from build123d import *

# Parameters (mm, degrees)
CROQUIS1_W              = 64
CROQUIS1_H              = 64
SALIENTE_EXTRUIR1_DEPTH = 60
CROQUIS2_W              = 70
CROQUIS2_H              = 70
CROQUIS2_W_2            = 64
CROQUIS2_H_2            = 64
SALIENTE_EXTRUIR2_DEPTH = 64
CORTAR_EXTRUIR1_DEPTH   = 21
CROQUIS5_R              = 1.1
CORTAR_EXTRUIR2_DEPTH   = 10
CORTAR_EXTRUIR3_REACH   = 30
CROQUIS10_R             = 4.5
CROQUIS11_W             = 70
CROQUIS11_H             = 70
CORTAR_EXTRUIR4_DEPTH   = 30
CROQUIS12_W             = 23
CROQUIS12_H             = 12.2
CORTAR_EXTRUIR5_DEPTH   = 21
CORTAR_EXTRUIR6_REACH   = 30
CROQUIS13_R             = 4.5
CROQUIS14_R             = 1.1
CORTAR_EXTRUIR7_DEPTH   = 10
CROQUIS15_R             = 3.7
CORTAR_EXTRUIR8_DEPTH   = 10
CROQUIS16_W             = 64
CROQUIS16_H             = 64
CORTAR_EXTRUIR9_DEPTH   = 5
CROQUIS17_W             = 12.5
CROQUIS17_H             = 12.998685397
CORTAR_EXTRUIR10_DEPTH  = 5
CORTAR_EXTRUIR11_REACH  = 72
CROQUIS18_W             = 70
CROQUIS18_H             = 9
CROQUIS18_H_2           = 5.000169364
CORTAR_EXTRUIR13_DEPTH  = 5
CORTAR_EXTRUIR14_REACH  = 12
CROQUIS21_W             = 81.467019472
CROQUIS21_H             = 81.467019472
CORTAR_EXTRUIR15_REACH  = 5
CROQUIS22_W             = 3.1
CROQUIS22_H             = 12.2


with BuildPart() as part:
    # Croquis1 → Saliente-Extruir1 (new body)
    with BuildSketch(Plane(origin=(0, 0, 0), x_dir=(1, 0, 0), z_dir=(0, 1, 0))):
        Rectangle(CROQUIS1_W, CROQUIS1_H)
    extrude(amount=SALIENTE_EXTRUIR1_DEPTH)

    # Croquis2 → Saliente-Extruir2 (add)
    with BuildSketch(Plane(origin=(0, 0, 0), x_dir=(1, 0, 0), z_dir=(0, 1, 0))):
        Rectangle(CROQUIS2_W, CROQUIS2_H)
        Rectangle(CROQUIS2_W_2, CROQUIS2_H_2, mode=Mode.SUBTRACT)
    extrude(amount=SALIENTE_EXTRUIR2_DEPTH)

    # Croquis4 → Cortar-Extruir1 (cut)
    with BuildSketch(Plane(origin=(0, 60, 0), x_dir=(1, 0, 0), z_dir=(0, 1, 0))):
        Polygon((-7, 6), (-7, -6), (-7, -6.25), (16, -6.25), (16, -6), (16, 6), (16, 6.25), (-7, 6.25), align=None)
    extrude(amount=-CORTAR_EXTRUIR1_DEPTH, mode=Mode.SUBTRACT)

    # Croquis5 → Cortar-Extruir2 (cut)
    with BuildSketch(Plane(origin=(0, 60, 0), x_dir=(1, 0, 0), z_dir=(0, 1, 0))):
        with Locations((19, 0)):
            Circle(CROQUIS5_R)
        with Locations((-9, 0)):
            Circle(CROQUIS5_R)
    extrude(amount=-CORTAR_EXTRUIR2_DEPTH, mode=Mode.SUBTRACT)

    # Croquis10 → Cortar-Extruir3 (cut, up to next)
    with BuildSketch(Plane(origin=(-7, 0, 0), x_dir=(0, 0, -1), z_dir=(1, 0, 0)), mode=Mode.PRIVATE) as cortar_extruir3_sk1:
        with Locations((0, 44)):
            Circle(CROQUIS10_R)
    cortar_extruir3_tool1 = extrude(cortar_extruir3_sk1.sketch, amount=-CORTAR_EXTRUIR3_REACH, mode=Mode.PRIVATE) & part.part
    add(cortar_extruir3_tool1.solids().sort_by_distance((-7, 44, 0))[0], mode=Mode.SUBTRACT)

    # Croquis11 → Cortar-Extruir4 (cut)
    with BuildSketch(Plane.XZ):
        Rectangle(CROQUIS11_W, CROQUIS11_H)
    extrude(amount=-CORTAR_EXTRUIR4_DEPTH, mode=Mode.SUBTRACT)

    # Croquis12 → Cortar-Extruir5 (cut)
    with BuildSketch(Plane.XZ.offset(-30)):
        with Locations((4.5, 22.1)):
            Rectangle(CROQUIS12_W, CROQUIS12_H)
    extrude(amount=-CORTAR_EXTRUIR5_DEPTH, mode=Mode.SUBTRACT)

    # Croquis13 → Cortar-Extruir6 (cut, up to next)
    with BuildSketch(Plane(origin=(-7, 0, 0), x_dir=(0, 0, -1), z_dir=(1, 0, 0)), mode=Mode.PRIVATE) as cortar_extruir6_sk1:
        with Locations((-22.1, 46)):
            Circle(CROQUIS13_R)
    cortar_extruir6_tool1 = extrude(cortar_extruir6_sk1.sketch, amount=-CORTAR_EXTRUIR6_REACH, mode=Mode.PRIVATE) & part.part
    add(cortar_extruir6_tool1.solids().sort_by_distance((-7, 46, 22.1))[0], mode=Mode.SUBTRACT)

    # Croquis14 → Cortar-Extruir7 (cut)
    with BuildSketch(Plane.XZ.offset(-30)):
        with Locations((19, 22.1)):
            Circle(CROQUIS14_R)
        with Locations((-9, 22.1)):
            Circle(CROQUIS14_R)
    extrude(amount=-CORTAR_EXTRUIR7_DEPTH, mode=Mode.SUBTRACT)

    # Croquis15 → Cortar-Extruir8 (cut)
    with BuildSketch(Plane.XZ.offset(-30)):
        with Locations((0, -22.1)):
            Circle(CROQUIS15_R)
    extrude(amount=-CORTAR_EXTRUIR8_DEPTH, mode=Mode.SUBTRACT)

    # Croquis16 → Cortar-Extruir9 (cut)
    with BuildSketch(Plane(origin=(0, 60, 0), x_dir=(1, 0, 0), z_dir=(0, 1, 0))):
        Rectangle(CROQUIS16_W, CROQUIS16_H)
    extrude(amount=-CORTAR_EXTRUIR9_DEPTH, mode=Mode.SUBTRACT)

    # Croquis17 → Cortar-Extruir10 (cut)
    with BuildSketch(Plane(origin=(-7, 0, 0), x_dir=(0, 0, -1), z_dir=(1, 0, 0))):
        with Locations((0, 45.499342699)):
            Rectangle(CROQUIS17_W, CROQUIS17_H)
    extrude(amount=-CORTAR_EXTRUIR10_DEPTH, mode=Mode.SUBTRACT)

    # Croquis18 → Cortar-Extruir11 (cut, up to next)
    with BuildSketch(Plane(origin=(35, 0, 0), x_dir=(0, 0, -1), z_dir=(1, 0, 0)), mode=Mode.PRIVATE) as cortar_extruir11_sk1:
        with Locations((0, 59.5)):
            Rectangle(CROQUIS18_W, CROQUIS18_H)
    cortar_extruir11_tool1 = extrude(cortar_extruir11_sk1.sketch, amount=-CORTAR_EXTRUIR11_REACH, mode=Mode.PRIVATE) & part.part
    add(cortar_extruir11_tool1.solids().sort_by_distance((35, 59.5, 0))[0], mode=Mode.SUBTRACT)
    # Croquis18 → Cortar-Extruir11 (cut, up to next)
    with BuildSketch(Plane(origin=(35, 0, 0), x_dir=(0, 0, -1), z_dir=(1, 0, 0)), mode=Mode.PRIVATE) as cortar_extruir11_sk2:
        with Locations((0, 32.500084682)):
            Rectangle(CROQUIS18_W, CROQUIS18_H_2)
    cortar_extruir11_tool2 = extrude(cortar_extruir11_sk2.sketch, amount=-CORTAR_EXTRUIR11_REACH, mode=Mode.PRIVATE) & part.part
    add(cortar_extruir11_tool2.solids().sort_by_distance((35, 32.500085, 0))[0], mode=Mode.SUBTRACT)

    # Croquis19 → Cortar-Extruir13 (cut)
    with BuildSketch(Plane(origin=(-7, 0, 0), x_dir=(0, 0, -1), z_dir=(1, 0, 0))):
        Polygon((-16, 51), (-28.2, 51), (-28.2, 38.000169364), (-22.1, 38.000169364), (-16, 38.000169364), align=None)
    extrude(amount=-CORTAR_EXTRUIR13_DEPTH, mode=Mode.SUBTRACT)

    # Croquis21 → Cortar-Extruir14 (cut, up to next)
    with BuildSketch(Plane(origin=(0, 45.000169364, 0), x_dir=(-1, 0, 0), z_dir=(0, -1, 0)), mode=Mode.PRIVATE) as cortar_extruir14_sk1:
        with Locations((0.076423095, -0.764230952)):
            Rectangle(CROQUIS21_W, CROQUIS21_H)
    cortar_extruir14_tool1 = extrude(cortar_extruir14_sk1.sketch, amount=-CORTAR_EXTRUIR14_REACH, mode=Mode.PRIVATE) & part.part
    add(cortar_extruir14_tool1.solids().sort_by_distance((-0.076423, 45.000169, 0.764231))[0], mode=Mode.SUBTRACT)

    # Croquis22 → Cortar-Extruir15 (cut, up to next)
    with BuildSketch(Plane(origin=(0, 38.000169364, 0), x_dir=(1, 0, 0), z_dir=(0, 1, 0)), mode=Mode.PRIVATE) as cortar_extruir15_sk1:
        with Locations((-8.55, -22.1)):
            Rectangle(CROQUIS22_W, CROQUIS22_H)
    cortar_extruir15_tool1 = extrude(cortar_extruir15_sk1.sketch, amount=-CORTAR_EXTRUIR15_REACH, mode=Mode.PRIVATE) & part.part
    add(cortar_extruir15_tool1.solids().sort_by_distance((-8.55, 38.000169, 22.1))[0], mode=Mode.SUBTRACT)


solid = part.part
Check sheet for the modelled part. Datum: model origin and axes. Units: mm. A direction names the side the tool comes from. Give positions to 0.01 mm unless a question says otherwise; leave off trailing zeros. Write each loop counter-clockwise with the first axis right and the second up, starting at its lowest first coordinate (ties: lowest second). Pieces come first, ordered by that corner, then holes. Notation, with made-up numbers: (78, 48) -> (84, 48) arc R38 cw to (84, 87) -> close; hole circle Ø11 at (14, 39.5). An arc over 180 degrees is marked (long way). One line per item, written item: value. Start each with the question number.
Item 1: Tool access check on faces 1 (the cylindrical face through (1.99, 37.47, -18.98)), 2 (the flat face through (2, 42, 6.25)), 3 (the flat face through (16, 40, 22)). Record the directions out of +Z, -Z, +X, -X, +Y, -Y that give a thin tool (end or side, any length) a straight path to the whole face; none if there is none.
Item 2: Draft check along Z on faces 4 (the flat face through (-11, 38, 22)), 5 (the flat face through (0, 40, -35)), 6 (the flat face through (0, 40, 35)). Enter one of: +Z half, -Z half, draft (parallel to the pull), parting line (faces both ways), or undercut.
Item 3: Section check C-C on z = 25.5. Record the cut outline in (x, y), then the cut area to 3 significant figures.
Item 4: Section check A-A on x = 11.5. Record the cut outline in (y, z).
Item 5: Section check B-B on y = 36.75. Record the cut outline in (x, z), then the cut area to 3 significant figures.
Item 6: Material ranges on probe 1 along Z at (x, y) = (3, 41.25); probe 2 along X at (y, z) = (42, -6); probe 3 along Z at (x, y) = (-21, 44), recorded low to high. Write a range as from..to.
Item 7: Gauge pin test, flat ends, axial feed: pin 1 (3 mm diameter, centred on x = 2, z = 0.5, fed in from +Y); pin 2 (0.9 mm diameter, centred on x = -11.5, z = 23.5, fed in from +Y). Record the tip position at first contact, or that the pin passes through.
Item 8: Section check D-D on x = 19. Record the cut outline in (y, z), then the cut area to 3 significant figures.
Results list:
1. face 1: -Y
1. face 2: +Y
1. face 3: +Y, -Y
2. face 4: undercut
2. face 5: -Z half
2. face 6: +Z half
3. outline: (-35, 35) -> (-10.1, 35) -> (-10.1, 38) -> (-12, 38) -> (-12, 43.05) -> (-35, 43.05) -> close; (16, 35) -> (35, 35) -> (35, 45) -> (16, 45) -> close
3. area: 381 mm²
4. outline: (35, -35) -> (45, -35) -> (45, -6.25) -> (39, -6.25) -> (39, 6.25) -> (45, 6.25) -> (45, 16) -> (35, 16) -> close; (35, 28.2) -> (45, 28.2) -> (45, 35) -> (35, 35) -> close
5. outline: (-35, -35) -> (35, -35) -> (35, 35) -> (-35, 35) -> close; hole (-10.1, 16) -> (16, 16) -> (16, 28.2) -> (-10.1, 28.2) -> close; hole circle Ø7.4 at (0, -22.1); hole circle Ø2.2 at (19, 22.1)
5. area: 4,530 mm²
6. probe 1: -35..-6.25, 6.25..16, 28.2..35
6. probe 2: -35..-12, 16..35
6. probe 3: -35..-4.5, 4.5..18.07, 26.13..35
7. pin 1: y = 39
7. pin 2: y = 38
8. outline: (35, -35) -> (45, -35) -> (45, 35) -> (35, 35) -> (35, 23.2) -> (40, 23.2) -> (40, 21) -> (35, 21) -> close
8. area: 689 mm²
